Can you work these out from the model? Positions are in its coordinate system, mm. A direction names the side the tool comes from. Round coordinates to 2 decimals unless told otherwise and drop trailing zeros. Order: outer loops, then holes, each group sorted by start corner. A loop starts at its lowest first (then second) coordinate and runs counter-clockwise, first axis right, second up. Notation, with made-up numbers: (42.5, 54) - (51.5, 54) arc R29 cw to (51.5, 91) - close; hole circle Ø10 at (52, -1). An arc over 180 degrees is marked (long way). Write item = value, one per line.
from build123d import *

# Parameters (mm, degrees)
CROQUIS2_R              = 13.875
CROQUIS2_R_2            = 10.7
SALIENTE_EXTRUIR1_START = -22.5
CROQUIS3_R              = 10.7
CROQUIS3_R_2            = 10.003405024
SALIENTE_EXTRUIR1_DEPTH = 1
SALIENTE_EXTRUIR2_START = -22.5
CROQUIS5_R              = 10.7
CROQUIS5_R_2            = 9.69715728
SALIENTE_EXTRUIR2_DEPTH = 1
SALIENTE_EXTRUIR3_START = 14
CROQUIS6_R              = 3.466635683
SALIENTE_EXTRUIR3_DEPTH = 1


with BuildPart() as part:
    # Barrer1: sweep along a path in Croquis1
    with BuildLine(Plane(origin=(0, 0, 0), x_dir=(1, 0, 0), z_dir=(0, 1, 0))) as barrer1_path:
        Line((-36.125, 0), (-14.5, 0))
        ThreePointArc((-14.5, 0), (-4.246951673, -4.246951673), (0, -14.5))
        Line((0, -14.5), (0, -36.125))
    # Croquis2 → Barrer1 (sweep)
    with BuildSketch(Plane.XY.offset(36.125)):
        Circle(CROQUIS2_R)
        Circle(CROQUIS2_R_2, mode=Mode.SUBTRACT)
    sweep(path=barrer1_path.line)

    # Croquis3 → Saliente-Extruir1 (add)
    with BuildSketch(Plane.XY.offset(36.125).offset(SALIENTE_EXTRUIR1_START)):
        Circle(CROQUIS3_R)
        Circle(CROQUIS3_R_2, mode=Mode.SUBTRACT)
    extrude(amount=-SALIENTE_EXTRUIR1_DEPTH)

    # Croquis5 → Saliente-Extruir2 (add)
    with BuildSketch(Plane.ZY.offset(36.125).offset(SALIENTE_EXTRUIR2_START)):
        Circle(CROQUIS5_R)
        Circle(CROQUIS5_R_2, mode=Mode.SUBTRACT)
    extrude(amount=SALIENTE_EXTRUIR2_DEPTH)

    # Croquis6 → Saliente-Extruir3 (add)
    with BuildSketch(Plane(origin=(0, 0, 0), x_dir=(1, 0, 0), z_dir=(0, 1, 0)).offset(SALIENTE_EXTRUIR3_START)):
        with Locations((0, -26.109260765)):
            Circle(CROQUIS6_R)
    extrude(amount=-SALIENTE_EXTRUIR3_DEPTH)


solid = part.part
(1) If I drill on line 1 (Y direction, x = 0, z = 13); line 2 (Y direction, x = -26, z = 0) (3 decimals); line 3 (X direction, y = 8.25, z = 22.5), over which ranges is the centre line in solid material (lowest first)? Write a range as from..to.
Computed:
line_1 = -13.87..-10, 10..13.87
line_2 = -13.875..-10.7, 10.7..13.875
line_3 = -11.16..-6.81, 6.81..11.16
(2) If we section it at B-B (z = 31): Write out the boundary of the cut face in (x, y) (3 decimals).
Computed:
outline = circle Ø27.75 at (0, 0); hole circle Ø21.4 at (0, 0)
(3) Thinking about a two-plate mould opening in Z: for faces 1 (the face through (-36.125, 10.2, 4)), 2 (the face through (9.4, -3.9, 13.625)), 3 (the face through (-25.161, 4.168, -13.234)), 4 (the face through (-14.118, -8.603, 4.475)), which applies, +Z half, -Z half, draft (parallel to the pull), parting line (faces both ways), or undercut?
Computed:
face_1 = draft
face_2 = +Z half
face_3 = parting line
face_4 = undercut
(4) On a 3-axis mill with a long thin cutter (end or side, diameter ignored), from which of +Z, -Z, +X, -X, +Y, -Y can I reach the whole of each face in a straight line? I mean faces 5 (the face through (-14.625, 10, -2)), 6 (the face through (-13.625, 10, -2)), 7 (the face through (-2.32, -10.446, 25.464)), 8 (the face through (-2.56, 13.84, 23.77)). Say none if no direction works.
Computed:
face_5 = -X
face_6 = none
face_7 = +Z
face_8 = +Y
(5) If we section it at A-A (y = 0): State how many separate pieces and enclosed holes the cut face has, plus the area to 3 significant figures.
Computed:
separate_pieces = 3
enclosed_holes = 0
area = 423 mm^2
(6) Will these pins go through, and if not, where does the flat tip stop? P1, Ø2, axis at x = -13.5, z = 4, coming from the +Y side; P2, Ø12, axis at x = -26, z = 17.5, coming from the -Y side; P3, Ø4, axis at y = 8, z = 18.5, coming from the -X side.
Computed:
P1 = 13.56
P2 = -7.76
P3 = -12.51
